Part print with two shaded views. Sizes in mm from the minimum x, y, z corner. A direction names the side the tool comes from. Coordinates: 2 decimals unless noted, no trailing zeros. Loops run counter-clockwise (first coordinate to the right, second up) from the corner with the lowest first, then second, coordinate; pieces in that order, holes last.
Item 1: Cut at C-C (y = 2.75). List the corners of the cut face in (x, z), and give its area (3 significant figures).
Item 2: Cut at B-B (x = 7.5). List the corners of the cut face in (y, z) (3 decimals), and give its area (3 significant figures).
Item 3: Flat gauge pins, fed straight in: pin 1 (1.5 mm diameter, centred on x = 3.5, z = 10, fed in from -Y); pin 2 (1 mm diameter, centred on y = 6.5, z = 10.5, fed in from +X); pin 3 (4 mm diameter, centred on x = 6, z = 7.5, fed in from +Y); pin 4 (3 mm diameter, centred on y = 5.5, z = 10.5, fed in from -X). Where does each tip first touch, or does it go through?
Item 4: Cut at D-D (z = 3). List the corners of the cut face in (x, y), and give its area (3 significant figures).
Item 5: Mould opens along Z. For the marked faces 3, 4 and 5 say: released by +Z, released by -Z, zero draft, split by the parting line, or undercut.
Item 6: Drill centre lines: line 1 along X through (y, z) = (0.85, 7.5) (3 decimals); line 2 along Y through (x, z) = (9.75, 5); line 3 along Z through (x, y) = (4.75, 2.75). Where is each one in solid material? Low to high.
Item 7: 3-axis set-ups, long thin cutter, end or side, ignore diameter. For the marked faces 1 and 2: which of +Z, -Z, +X, -X, +Y, -Y reach the whole face in a straight line?
Item 8: Cut at A-A (z = 7.5). List the corners of the cut face in (x, y) (3 decimals).
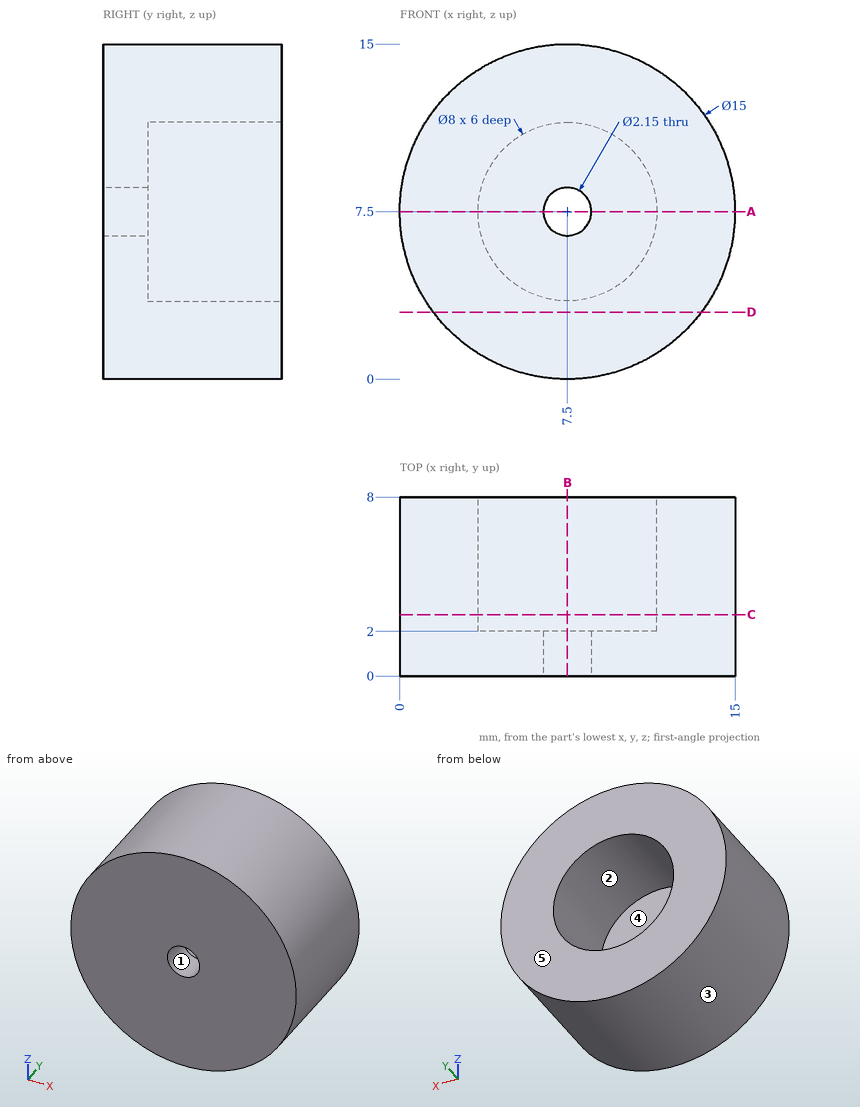
Filled sheet:
1. outline: circle Ø15 at (7.5, 7.5); hole circle Ø8 at (7.5, 7.5)
1. area: 126 mm2
2. outline: (0, 0) - (8, 0) - (8, 3.5) - (2, 3.5) - (2, 6.425) - (0, 6.425) - close; (0, 8.575) - (2, 8.575) - (2, 11.5) - (8, 11.5) - (8, 15) - (0, 15) - close
2. area: 67.7 mm2
3. pin 1: stops at y = 0
3. pin 2: stops at x = 14.57
3. pin 3: stops at y = 2
3. pin 4: stops at x = 0.15
4. outline: (1.5, 0) - (13.5, 0) - (13.5, 8) - (1.5, 8) - close
4. area: 96.0 mm2
5. face 3: split by the parting line
5. face 4: undercut
5. face 5: zero draft
6. line 1: x = 0 to 6.425, 8.575 to 15
6. line 2: y = 0 to 2
6. line 3: z = 0.52 to 4.6, 10.4 to 14.48
7. face 1: +Y, -Y
7. face 2: +Y
8. outline: (0, 0) - (6.425, 0) - (6.425, 2) - (3.5, 2) - (3.5, 8) - (0, 8) - close; (8.575, 0) - (15, 0) - (15, 8) - (11.5, 8) - (11.5, 2) - (8.575, 2) - close
